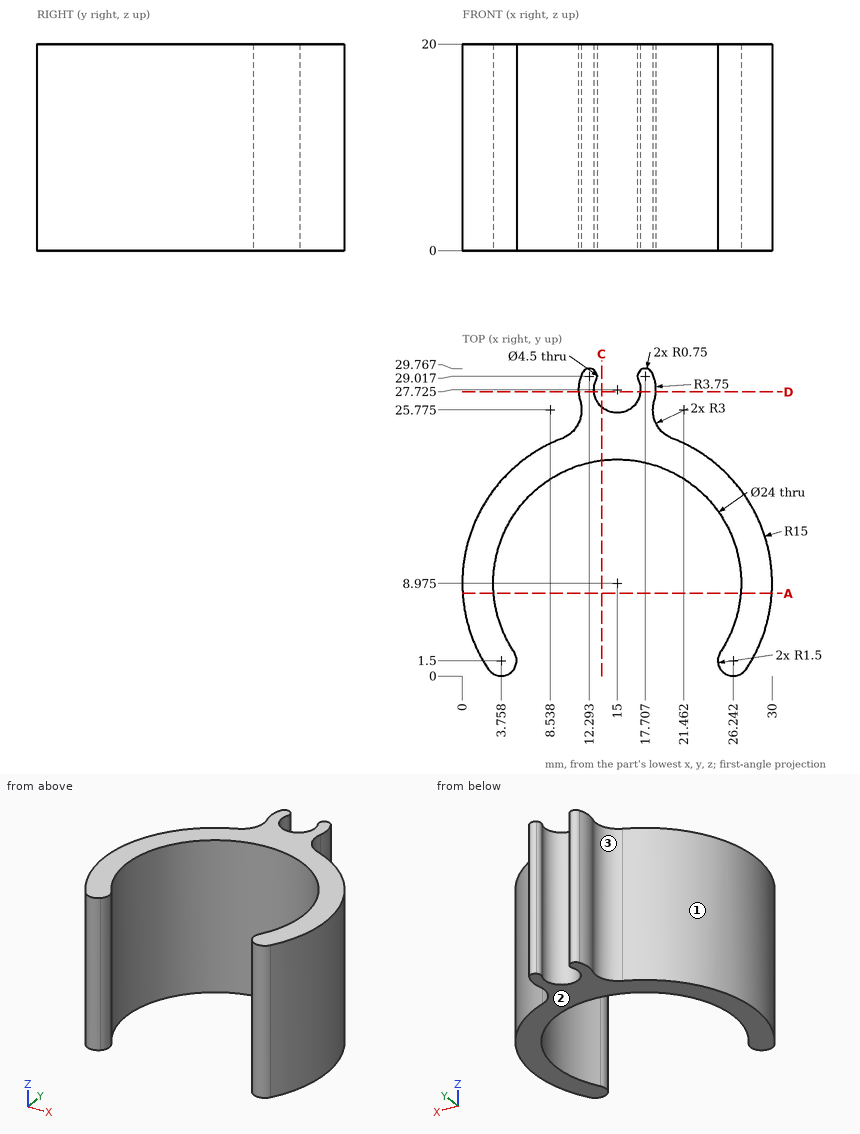
Study the drawing (mm; zero at the part's minimum x, y, z) and answer. Coordinates: 2 decimals unless noted, no trailing zeros. Write each loop counter-clockwise with the first axis right and the second up, starting at its lowest first coordinate (ties: lowest second). Pieces come first, ordered by that corner, then holes.
Q1. Section D-D, the plane y = 27.5 is taken. Write down the section's boundary in (x, z).
Returned:
outline: (11.26, 0) - (12.76, 0) - (12.76, 20) - (11.26, 20) - close; (17.24, 0) - (18.74, 0) - (18.74, 20) - (17.24, 20) - close
Q2. Find the intervals of material crossed by line 1 along Y through (x, z) = (15, 15.25) (1 decimal); line 2 along X through (y, z) = (3, 8.75) (1 decimal); line 3 along X through (y, z) = (6, 15) (1 decimal), in increasing order.
Returned:
line 1: y = 21 to 25.5
line 2: x = 1.2 to 4.6, 25.4 to 28.8
line 3: x = 0.3 to 3.4, 26.6 to 29.7
Q3. Given P1, Ø12, axis at x = 10.5, z = 3, coming from the -Y side; P2, Ø10, axis at x = 11, z = 17.5, coming from the -Y side; P3, Ø3, axis at x = 5, z = 6.5, coming from the +Y side (1 decimal), each flat-ended and moving along its own axis, determine where each tip first touches the part or whether it passes through.
Returned:
P1: stops at y = 0.2
P2: stops at y = 16.91
P3: stops at y = 21.3
Q4. Section C-C, the plane x = 13.5 is taken. Write down the section's boundary in (y, z).
Returned:
outline: (20.88, 0) - (26.05, 0) - (26.05, 20) - (20.88, 20) - close
Q5. Section A-A, the plane y = 8 is taken. Write down the section's boundary in (x, z), then the cut area to 3 significant figures.
Returned:
outline: (0.03, 0) - (3.04, 0) - (3.04, 20) - (0.03, 20) - close; (26.96, 0) - (29.97, 0) - (29.97, 20) - (26.96, 20) - close
area: 120 mm2
Q6. The mould has two halves that part along Y. Classify the marked faces 1, 2 and 3: released by +Y, released by -Y, zero draft, split by the parting line, or undercut.
Returned:
face 1: split by the parting line
face 2: zero draft
face 3: undercut
